```python
from build123d import *

# Parameters (mm, degrees)
SKETCH1_R            = 227.325
SKETCH1_R_2          = 203.325
EXTRUDE1_DEPTH       = 4.7
SKETCH2_R            = 217.625
EXTRUDE2_DEPTH       = 322.520452304
M4_CLEARANCE_HOLE1_D = 4.5
CIRPATTERN1_COUNT    = 24
SKETCH11_R           = 2.25
SKETCH11_R_2         = 2
BOSS_EXTRUDE2_DEPTH  = 4.7
CHAMFER1_SIZE        = 2.1


with BuildPart() as part:
    # Sketch1 → Extrude1 (new body)
    with BuildSketch(Plane.XY):
        Circle(SKETCH1_R)
        Circle(SKETCH1_R_2, mode=Mode.SUBTRACT)
    extrude(amount=EXTRUDE1_DEPTH)

    # Sketch2 → Extrude2 (cut, through all)
    with BuildSketch(Plane(origin=(0, 0, 0), x_dir=(-1, 0, 0), z_dir=(0, 0, -1))):
        Circle(SKETCH2_R)
    extrude(amount=-EXTRUDE2_DEPTH, mode=Mode.SUBTRACT)

    # M4 Clearance Hole1 (through all)
    with Locations(Plane.XY.offset(4.7)):
        with Locations((0, 222)):
            m4_clearance_hole1 = Hole(M4_CLEARANCE_HOLE1_D / 2)

    # CirPattern1: M4 Clearance Hole1 ×24 about axis
    cirpattern1_axis = Axis((0, 0, 0), (0, 0, 1))
    for i in range(1, CIRPATTERN1_COUNT):
        add(m4_clearance_hole1.rotate(cirpattern1_axis, i * 360 / CIRPATTERN1_COUNT), mode=Mode.SUBTRACT)

    # Sketch11 → Boss-Extrude2 (add)
    with BuildSketch(Plane.XY.offset(4.7)):
        with Locations((222, 0)):
            Circle(SKETCH11_R)
        with Locations((222, 0)):
            Circle(SKETCH11_R_2, mode=Mode.SUBTRACT)
        with Locations((-222, 0)):
            Circle(SKETCH11_R)
        with Locations((-222, 0)):
            Circle(SKETCH11_R_2, mode=Mode.SUBTRACT)
    extrude(amount=-BOSS_EXTRUDE2_DEPTH)

    # Chamfer1
    chamfer1_edges = [part.edges().sort_by_distance(p)[0] for p in [
        (217.625, 0, 4.7),
    ]]
    chamfer(chamfer1_edges, length=CHAMFER1_SIZE)


solid = part.part
```
Input: part model. Units: mm. Frame: model coordinates. Coordinates: 2 decimals unless noted, no trailing zeros. Put each result on its own line as item: value.
1. Line query: line 1 along Y through (x, z) = (0, 3.25) (3 decimals); line 2 along X through (y, z) = (93, 4); line 3 along X through (y, z) = (-185.5, 0.7). Output: solid intervals per line, ascending.
Report:
line 1: y = -227.325 to -224.25, -219.75 to -218.275, 218.275 to 219.75, 224.25 to 227.325
line 2: x = -207.43 to -198.3, 198.3 to 207.43
line 3: x = -131.4 to -113.8, 113.8 to 131.4
2. Draft query along X for faces 1 (the face through (-119, 186, 4.7)), 2 (the face through (47.18, -212.45, 1.28)), 3 (the face through (-49.28, -221.92, 2.32)). Return one class per face: pulls with the +X half, pulls with the -X half, needs draft (parallel to the pull), parting line crosses it, or undercut.
Report:
face 1: needs draft
face 2: undercut
face 3: parting line crosses it
3. Contact query for a flat-ended pin moving along its axis: pin 1 Ø4 at (x, y) = (0, -222) entering from +Z. Output: stop coordinate, or through.
Report:
pin 1: passes through
4. Cut plane A-A on z = 3.85. State how many separate pieces and enclosed holes the cut face has, then the cut area to 3 significant figures.
Report:
separate pieces: 1
enclosed holes: 25
area: 11,500 mm2
